Autodesk Inventor part; units mm, degrees
ref_plane "YZ Plane" through (0, 0, 0) normal (1, 0, 0) x (0, 1, 0)
ref_plane "XZ Plane" through (0, 0, 0) normal (0, 1, 0) x (-1, 0, 0)
ref_plane "XY Plane" through (0, 0, 0) normal (0, 0, 1) x (1, 0, 0)
sketch "Sketch1" plane through (0, 0, 0) normal (1, 0, 0) x (0, 1, 0)
  line L0 (-9, 13) -> (-9, 0)
  line L1 (-9, 0) -> (9, 0)
  line L2 (9, 0) -> (9, 4)
  line L3 (9, 4) -> (5, 13)
  line L4 (5, 13) -> (-9, 13)
  point P0 (0, 0)
  dimension "d0" = 13
  dimension "d1" = 18
  dimension "d2" = 9
  dimension "d3" = 0
  dimension "d4" = 4
  dimension "d5" = 14
extrude "Extrusion1" add sketch "Sketch1" along normal blind 14
sketch "Sketch2" plane through (0, -9, 0) normal (0, -1, 0) x (1, 0, 0)
  line L0 (0, 13) -> (0, 0)
  line L1 (14, 13) -> (14, 0)
  line L2 (0, 13) -> (14, 13)
  line L3 (2, 11) -> (12, 11)
  line L4 (12, 11) -> (12, 4)
  line L5 (12, 4) -> (2, 4)
  line L6 (2, 4) -> (2, 11)
  line L7 (3.5, 2) -> (10.5, 2)
  line L8 (10.5, 2) -> (10.5, 4)
  line L9 (10.5, 4) -> (3.5, 4)
  line L10 (3.5, 4) -> (3.5, 2)
  dimension "d8" = 10
  dimension "d9" = 7
  dimension "d10" = 2
  dimension "d11" = 2
  dimension "d12" = 2
  dimension "d13" = 7
  dimension "d14" = 2
  dimension "d15" = 0
  dimension "d16" = 3.5
extrude "Extrusion2" cut sketch "Sketch2" against normal blind 10
sketch "Sketch3" plane through (0, -9, 0) normal (0, 0, -1) x (-1, 0, 0)
  line L0 (0, 0) -> (0, 18)
  line L1 (-14, 0) -> (-14, 18)
  line L2 (0, 0) -> (-14, 0)
  circle A0 centre (-12.5, 8) radius 1.5
  circle A1 centre (-1.5, 8) radius 1.5
  point P0 (0, 9)
  dimension "d19" = 3
  dimension "d20" = 1.5
  dimension "d21" = 1.5
  dimension "d22" = 8
  dimension "d23" = 8
extrude "Extrusion3" add sketch "Sketch3" along normal blind 4
equation "\"d11\" = d12"
properties part number "6P6C" material "PC/ABS Plastic"
Work out the finished part from the listing and answer in its coordinate system (mm). A direction names the side the tool comes from. Give positions to 0.01 mm unless a question says otherwise; leave off trailing zeros. Write each loop counter-clockwise with the first axis right and the second up, starting at its lowest first coordinate (ties: lowest second). Pieces come first, ordered by that corner, then holes. Notation, with made-up numbers: (52.5, 48) - (91.5, 48) arc R22 cw to (91.5, 54) - close; hole circle Ø9 at (25, 45.5). An arc over 180 degrees is marked (long way). Use one line per item in the form item = value.
1. A cutting plane is placed at B-B (x = 1.5). Write down the section's boundary in (y, z), and give its area (3 significant figures).
Filled in:
outline = (-9, 0) - (-2.5, 0) - (-2.5, -4) - (0.5, -4) - (0.5, 0) - (9, 0) - (9, 4) - (5, 13) - (-9, 13) - close
area = 228 mm^2
2. A cutting plane is placed at C-C (z = -1.5). Write down the section's boundary in (x, y).
Filled in:
outline = circle Ø3 at (1.5, -1); circle Ø3 at (12.5, -1)
3. Each of these flat-tipped pins is pushed along its axis until it touches: pin 1 Ø7 at (x, z) = (8.5, 4.5) entering from -Y; pin 2 Ø3 at (x, y) = (5.5, -5.5) entering from -Z. Where does it stop, or does it pass through?
Filled in:
pin_1 = -9
pin_2 = 0
4. For faces 5 (the face through (14, 0, 7)), 6 (the face through (14, -1, -2)), 7 (the face through (3, -4, 4)), determine the directions among +Z, -Z, +X, -X, +Y, -Y from which every point of the face is accessible in a straight line to the end or side of a thin tool.
Filled in:
face_5 = +Z, -Z, +X, +Y, -Y
face_6 = -Z
face_7 = -Y
5. A cutting plane is placed at D-D (z = 3). Write down the section's boundary in (x, y).
Filled in:
outline = (0, -9) - (3.5, -9) - (3.5, 1) - (10.5, 1) - (10.5, -9) - (14, -9) - (14, 9) - (0, 9) - close
6. Consider L1, parallel to Z at x = 8.75, y = -7.5; L2, parallel to X at y = -6.5, z = 8; L3, parallel to Z at x = 1, y = -4. Determine where each line is inside the solid, lowest interval first.
Filled in:
L1 = 0 to 2, 11 to 13
L2 = 0 to 2, 12 to 14
L3 = 0 to 13
7. A cutting plane is placed at A-A (y = -7.25). Write down the section's boundary in (x, z).
Filled in:
outline = (0, 0) - (14, 0) - (14, 13) - (0, 13) - close; hole (2, 4) - (3.5, 4) - (3.5, 2) - (10.5, 2) - (10.5, 4) - (12, 4) - (12, 11) - (2, 11) - close
8. Determine the mould class of faces 1 (the face through (7, -2, 13)), 2 (the face through (3.5, -4, 3)), 3 (the face through (7, 0, 0)), 4 (the face through (0, 0, 7)) for opening direction X: released by +X, released by -X, zero draft, split by the parting line, or undercut.
Filled in:
face_1 = zero draft
face_2 = undercut
face_3 = undercut
face_4 = released by -X
